from build123d import *

# Parameters (mm, degrees)
BOX002_W     = 30
BOX002_H     = 16.5
BOX002_DEPTH = 11
BOX001_W     = 30
BOX001_H     = 16.5
BOX001_DEPTH = 3
BOX_W        = 97
BOX_H        = 100
BOX_DEPTH    = 3
BOX028_W     = 9
BOX028_H     = 10
BOX028_DEPTH = 3
BOX027_W     = 9
BOX027_H     = 7
BOX027_DEPTH = 3
BOX026_W     = 9
BOX026_H     = 10
BOX026_DEPTH = 3
BOX008_W     = 9
BOX008_H     = 10
BOX008_DEPTH = 3
BOX010_W     = 9
BOX010_H     = 7
BOX010_DEPTH = 3
BOX005_W     = 9
BOX005_H     = 10
BOX005_DEPTH = 3
BOX003_W     = 3
BOX003_H     = 67
BOX003_DEPTH = 47


with BuildPart() as obj1:
    # Box002 → Box002 (new body)
    with BuildSketch(Plane(origin=(67, 83.5, -4), x_dir=(1, 0, 0), z_dir=(0, 0, 1))):
        with Locations((15, 8.25)):
            Rectangle(BOX002_W, BOX002_H)
    extrude(amount=BOX002_DEPTH)


with BuildPart() as obj2:
    # Box001 → Box001 (new body)
    with BuildSketch(Plane(origin=(67, 0, 0), x_dir=(1, 0, 0), z_dir=(0, 0, 1))):
        with Locations((15, 8.25)):
            Rectangle(BOX001_W, BOX001_H)
    extrude(amount=BOX001_DEPTH)


with BuildPart() as base_con_agujeros_rueda:
    # Box → Box (new body)
    with BuildSketch(Plane.XY):
        with Locations((48.5, 50)):
            Rectangle(BOX_W, BOX_H)
    extrude(amount=BOX_DEPTH)

    # Cut: cut obj2
    add(obj2.part, mode=Mode.SUBTRACT)

    # Cut001: cut obj1
    add(obj1.part, mode=Mode.SUBTRACT)


with BuildPart() as box028:
    # Box028 → Box028 (new body)
    with BuildSketch(Plane(origin=(94, 63.5, 22), x_dir=(1, 0, 0), z_dir=(0, 0, 1))):
        with Locations((4.5, 5)):
            Rectangle(BOX028_W, BOX028_H)
    extrude(amount=BOX028_DEPTH)


with BuildPart() as centro002:
    # Box027 → Box027 (new body)
    with BuildSketch(Plane(origin=(94, 46.5, 22), x_dir=(1, 0, 0), z_dir=(0, 0, 1))):
        with Locations((4.5, 3.5)):
            Rectangle(BOX027_W, BOX027_H)
    extrude(amount=BOX027_DEPTH)


with BuildPart() as box026:
    # Box026 → Box026 (new body)
    with BuildSketch(Plane(origin=(94, 26.5, 22), x_dir=(1, 0, 0), z_dir=(0, 0, 1))):
        with Locations((4.5, 5)):
            Rectangle(BOX026_W, BOX026_H)
    extrude(amount=BOX026_DEPTH)


with BuildPart() as box008:
    # Box008 → Box008 (new body)
    with BuildSketch(Plane(origin=(91, 63.5, 44), x_dir=(1, 0, 0), z_dir=(0, 0, 1))):
        with Locations((4.5, 5)):
            Rectangle(BOX008_W, BOX008_H)
    extrude(amount=BOX008_DEPTH)


with BuildPart() as centro:
    # Box010 → Box010 (new body)
    with BuildSketch(Plane(origin=(91, 46.5, 44), x_dir=(1, 0, 0), z_dir=(0, 0, 1))):
        with Locations((4.5, 3.5)):
            Rectangle(BOX010_W, BOX010_H)
    extrude(amount=BOX010_DEPTH)


with BuildPart() as box005:
    # Box005 → Box005 (new body)
    with BuildSketch(Plane(origin=(91, 26.5, 44), x_dir=(1, 0, 0), z_dir=(0, 0, 1))):
        with Locations((4.5, 5)):
            Rectangle(BOX005_W, BOX005_H)
    extrude(amount=BOX005_DEPTH)


with BuildPart() as obj3:
    # Box003 → Box003 (new body)
    with BuildSketch(Plane(origin=(94, 16.5, 0), x_dir=(1, 0, 0), z_dir=(0, 0, 1))):
        with Locations((1.5, 33.5)):
            Rectangle(BOX003_W, BOX003_H)
    extrude(amount=BOX003_DEPTH)

    # Cut002: cut Box005
    add(box005.part, mode=Mode.SUBTRACT)

    # Cut003: cut centro
    add(centro.part, mode=Mode.SUBTRACT)

    # Cut004: cut Box008
    add(box008.part, mode=Mode.SUBTRACT)

    # Cut015: cut Box026
    add(box026.part, mode=Mode.SUBTRACT)

    # Cut016: cut centro002
    add(centro002.part, mode=Mode.SUBTRACT)

    # Cut017: cut Box028
    add(box028.part, mode=Mode.SUBTRACT)

    # Fusion004: union base con agujeros rueda
    add(base_con_agujeros_rueda.part)


solid = obj3.part
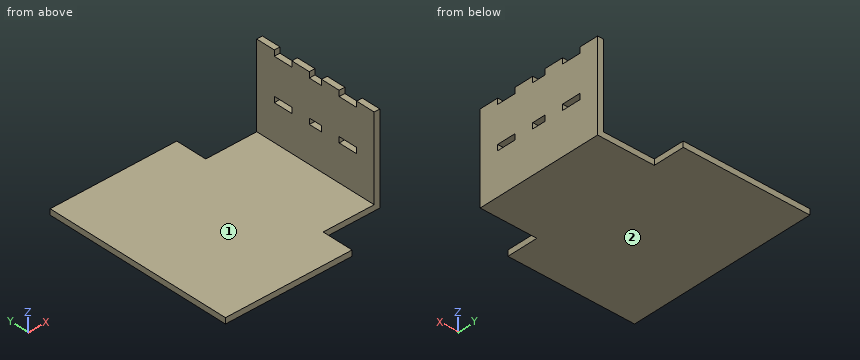
Here's how the part is built. I have some questions about the finished solid (model axes, mm). Face numbers are marked on the shaded views. A direction names the side the tool comes from. Round coordinates to 2 decimals unless told otherwise and drop trailing zeros. Order: outer loops, then holes, each group sorted by start corner. A loop starts at its lowest first (then second) coordinate and runs counter-clockwise, first axis right, second up. Notation, with made-up numbers: M -22,-40 L 21,-40 A13 ccw 21,-20 Z; hole C 23.5,40 d8. An arc over 180 degrees is marked long. Return JSON: item names as keys, results as strings. Group by question number.
1. If we section it at A-A on y = 29.5: List the corners of the cut face in (x, z) for me.
2. If we section it at D-D on z = 16: List the corners of the cut face in (x, y) for me.
3. On a 3-axis mill with a long thin cutter (end or side, diameter ignored), from which of +Z, -Z, +X, -X, +Y, -Y can I reach the whole of each face in a straight line? I mean the marked faces 1 and 2. Say none if no direction works.
4. I'm going to push flat-ended pins straight in: pin 1 Ø2.5 at (x, y) = (95.5, 48.5) entering from +Z; pin 2 Ø2.5 at (x, z) = (96, 23) entering from +Y; pin 3 Ø3.5 at (x, z) = (95, 45.5) entering from -Y; pin 4 Ø2.5 at (x, y) = (95.5, 33.5) entering from -Z. Where does each tip first touch, or does it pass through?
5. If we section it at C-C on x = 75.5: List the corners of the cut face in (y, z) for me, then the cut area to 3 significant figures.
6. If we section it at B-B on y = 42.5: List the corners of the cut face in (x, z) for me, then the cut area to 3 significant figures.
7. Please list where these lines run through material, in increasing order: probe 1 along Z at (x, y) = (26, 25); probe 2 along X at (y, z) = (66, 11.5).
Reply:
{
 "1": {"outline": "M 0,0 L 97,0 L 97,22 L 94,22 L 94,3 L 0,3 Z; M 94,25 L 97,25 L 97,44 L 94,44 Z"},
 "2": {"outline": "M 94,16.5 L 97,16.5 L 97,83.5 L 94,83.5 Z"},
 "3": {"face 1": "+Z, -X, +Y, -Y", "face 2": "-Z, +X, -X, +Y, -Y"},
 "4": {"pin 1": "z = 44", "pin 2": "y = 83.5", "pin 3": "y = 16.5", "pin 4": "z = 0"},
 "5": {"outline": "M 16.5,0 L 83.5,0 L 83.5,3 L 16.5,3 Z", "area": "201 mm^2"},
 "6": {"outline": "M 0,0 L 97,0 L 97,47 L 94,47 L 94,3 L 0,3 Z", "area": "423 mm^2"},
 "7": {"probe 1": "0 to 3", "probe 2": "94 to 97"}
}
